Geometry: see drawing. Coordinates: mm, zero at the bounding-box minimum. A direction names the side the tool comes from. Give positions to 0.01 mm unless a question says otherwise; leave off trailing zeros. Loops run counter-clockwise (first coordinate to the right, second up) from the corner with the lowest first, then second, coordinate; pieces in that order, holes last. Notation, with made-up numbers: M 61,48 L 90,48 A18 cw 90,79 Z; hole C 11.25,87 d4. An arc over 180 degrees is marked long. Use CSV: the item, a comma, the result in double quotes. Start each with the question number.
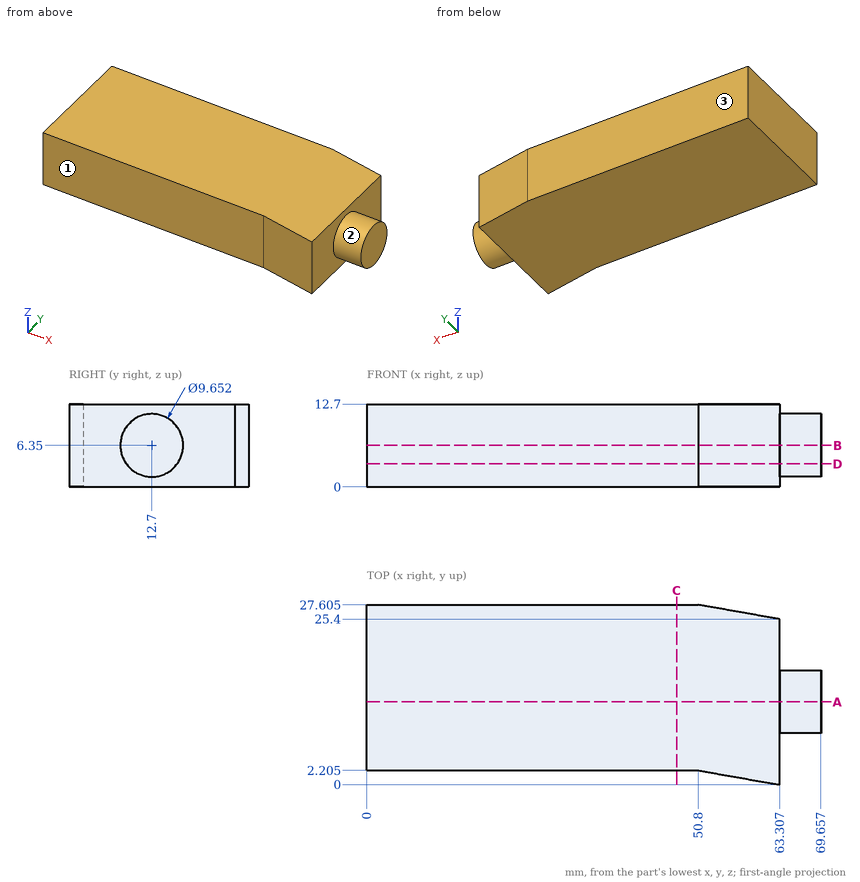
Item 1: Section A-A (y = 12.7). Output: boundary loops of the cut face in (x, z), then the cut area to 3 significant figures.
Item 2: Section C-C (x = 47.5). Output: boundary loops of the cut face in (y, z) (1 decimal), then the cut area to 3 significant figures.
Item 3: Section D-D (z = 3.5). Output: boundary loops of the cut face in (x, y) (1 decimal), then the cut area to 3 significant figures.
Item 4: First-contact query: pin 1 Ø3 at (y, z) = (18.5, 11.5) entering from +X; pin 2 Ø1.5 at (x, z) = (61, 4.5) entering from -Y (1 decimal); pin 3 Ø1.5 at (x, y) = (17.5, 17) entering from -Z; pin 4 Ø6.5 at (x, z) = (23, 8) entering from -Y (1 decimal). Flat tips, straight axial feed; report the tip coordinate or a pass-through.
Item 5: Material intervals for line 1 (X direction, y = 4.25, z = 4.5); line 2 (Y direction, x = 25, z = 7.25) (1 decimal); line 3 (Y direction, x = 60, z = 8.75), sorted ascending.
Item 6: Section B-B (z = 6.35). Output: boundary loops of the cut face in (x, y) (1 decimal).
Item 7: Set-up query: the marked faces 1, 2 and 3. Return all of +Z, -Z, +X, -X, +Y, -Y with unobstructed straight access to the full face (end or side cutting, diameter ignored); none if empty.
Recorded:
1,outline,"M 0,0 L 63.31,0 L 63.31,1.52 L 69.66,1.52 L 69.66,11.18 L 63.31,11.18 L 63.31,12.7 L 0,12.7 Z"
1,area,"865 mm²"
2,outline,"M 2.2,0 L 27.6,0 L 27.6,12.7 L 2.2,12.7 Z"
2,area,"323 mm²"
3,outline,"M 0,2.2 L 50.8,2.2 L 63.3,0 L 63.3,8.8 L 69.7,8.8 L 69.7,16.6 L 63.3,16.6 L 63.3,25.4 L 50.8,27.6 L 0,27.6 Z"
3,area,"1,660 mm²"
4,pin 1,"x = 63.31"
4,pin 2,"y = 0.3"
4,pin 3,"z = 0"
4,pin 4,"y = 2.2"
5,line 1,"0 to 63.31"
5,line 2,"2.2 to 27.6"
5,line 3,"0.58 to 25.98"
6,outline,"M 0,2.2 L 50.8,2.2 L 63.3,0 L 63.3,7.9 L 69.7,7.9 L 69.7,17.5 L 63.3,17.5 L 63.3,25.4 L 50.8,27.6 L 0,27.6 Z"
7,face 1,"+Z, -Z, -X, -Y"
7,face 2,"+X"
7,face 3,"+Z, -Z, +X, -X, +Y"
